The listing builds one solid part. Answer for the finished solid, in the listing's coordinates (mm). Face numbers are marked on the shaded views. A direction names the side the tool comes from. Round coordinates to 2 decimals unless told otherwise and drop trailing zeros. Write each loop counter-clockwise with the first axis right and the second up, starting at its lowest first coordinate (ties: lowest second). Pieces come first, ordered by that corner, then holes. Notation, with made-up numbers: M 65,45.5 L 110,45.5 A16 cw 110,59.5 Z; hole C 47.5,-33 d6. An arc over 180 degrees is marked long. Answer as CSV lines item,"result". Start each with the question number.
from build123d import *

# Parameters (mm, degrees)
SKETCH010_W  = 2.513972
SKETCH010_H  = 2.513972
PAD003_DEPTH = 1.5
PAD004_DEPTH = 1
SKETCH011_W  = 4.09222
SKETCH011_H  = 4.09222
PAD005_DEPTH = 3.5


with BuildPart() as part:
    # Sketch010 (on Face1 of ShapeBinder002) → Pad003 (new body)
    with BuildSketch(Plane.XY.offset(23.22)):
        with Locations((13.05, 9.55)):
            Rectangle(SKETCH010_W, SKETCH010_H)
    extrude(amount=PAD003_DEPTH)

    # Sketch010 (on Face1 of ShapeBinder002) → Pad004 (join)
    with BuildSketch(Plane.XY.offset(23.22)):
        with Locations((13.05, 9.55)):
            Rectangle(SKETCH010_W, SKETCH010_H)
    extrude(amount=-PAD004_DEPTH)

    # Sketch011 (on Face1 of Pad004) → Pad005 (join)
    with BuildSketch(Plane(origin=(0, 0, 22.22), x_dir=(1, 0, 0), z_dir=(0, 0, -1))):
        with Locations((13.05, -9.55)):
            Rectangle(SKETCH011_W, SKETCH011_H)
    extrude(amount=PAD005_DEPTH)


solid = part.part
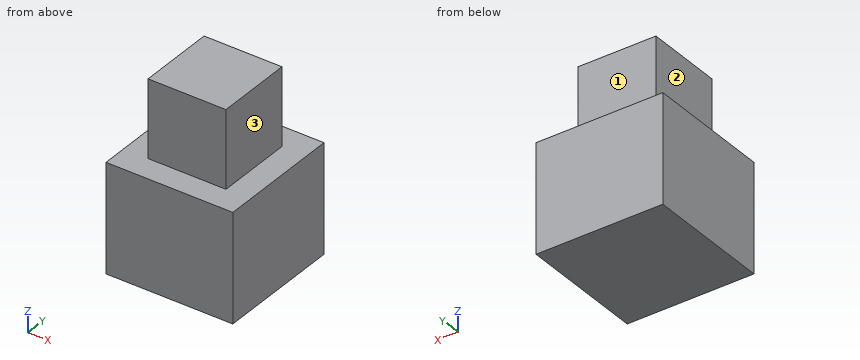
Q1. Each of these flat-tipped pins is pushed along its axis until it touches: P1, Ø1.2, axis at y = 9.5, z = 23, coming from the +X side; P2, Ø1.2, axis at x = 12.5, z = 23, coming from the -Y side. Where does it stop, or does it pass through?
Q2. Straight lines are drawn through the part: L1, parallel to Y at x = 13.7, z = 23.05; L2, parallel to Z at x = 11.6, y = 7.8; L3, parallel to X at y = 9.2, z = 23.9. For each, find the intervals that lie inside material, in ascending order.
Q3. Find section D-D (y = 11.1). Determine the outline of the cut face in (x, z).
Q4. Find section A-A (y = 9.5). Determine the outline of the cut face in (x, z).
Q5. Find section B-B (x = 12.15). Determine the outline of the cut face in (y, z), plus the area to 3 significant figures.
Q6. For the marked faces 1, 2 and 3, determine the directions among +Z, -Z, +X, -X, +Y, -Y from which every point of the face is accessible in a straight line to the end or side of a thin tool.
Q7. Find section C-C (z = 23.8). Determine the outline of the cut face in (x, y).
Reported:
1,P1,"stops at x = 14.31"
1,P2,"stops at y = 8.29"
2,L1,"y = 8.29 to 10.81"
2,L2,"z = 18.72 to 22.22"
2,L3,"x = 11.79 to 14.31"
3,outline,"M 11,18.72 L 15.1,18.72 L 15.1,22.22 L 11,22.22 Z"
4,outline,"M 11,18.72 L 15.1,18.72 L 15.1,22.22 L 14.31,22.22 L 14.31,24.72 L 11.79,24.72 L 11.79,22.22 L 11,22.22 Z"
5,outline,"M 7.5,18.72 L 11.6,18.72 L 11.6,22.22 L 10.81,22.22 L 10.81,24.72 L 8.29,24.72 L 8.29,22.22 L 7.5,22.22 Z"
5,area,"20.6 mm2"
6,face 1,"+Z, +X, -X, +Y"
6,face 2,"+Z, -X, +Y, -Y"
6,face 3,"+Z, +X, +Y, -Y"
7,outline,"M 11.79,8.29 L 14.31,8.29 L 14.31,10.81 L 11.79,10.81 Z"
